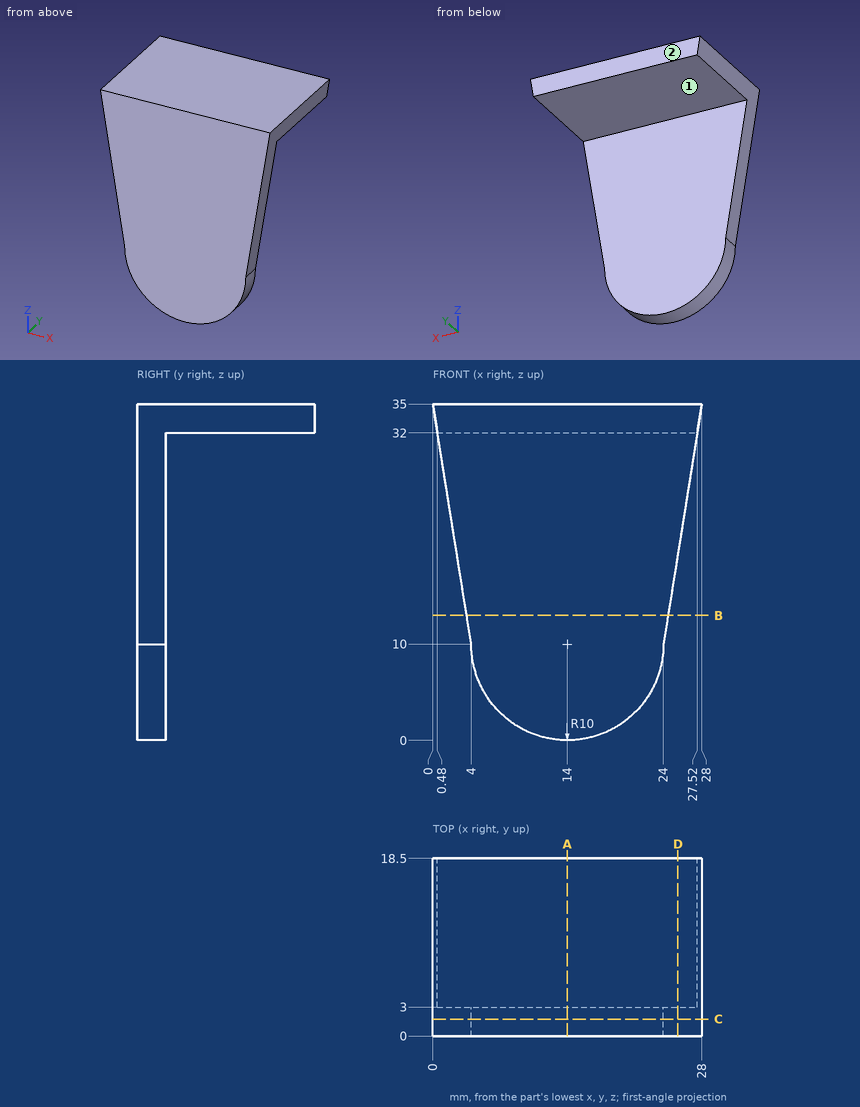
Source: three-view drawing plus pictorial views. Frame: mm from the lowest corner of the part. A direction names the side the tool comes from. Round coordinates to 2 decimals unless told otherwise and drop trailing zeros. Loops run counter-clockwise (first coordinate to the right, second up) from the corner with the lowest first, then second, coordinate; pieces in that order, holes last.
1. Ray query, L1, parallel to Z at x = 16.75, y = 5.75; L2, parallel to Y at x = 20.75, z = 3; L3, parallel to X at y = 1.75, z = 4.5. Return the intervals inside material, ascending.
2. Contact query for flat-ended pins moving along their axis: pin 1 (3 mm diameter, centred on x = 7, y = 6, fed in from -Z); pin 2 (8 mm diameter, centred on x = 12, z = 26.5, fed in from -Y); pin 3 (3 mm diameter, centred on x = 3.5, z = 19, fed in from +Y). Output: stop coordinate, or through.
3. Section query D-D on x = 25.5. Output: boundary loops of the cut face in (y, z) (3 decimals).
4. Access query for the marked faces 1 and 2. Directions: +Z, -Z, +X, -X, +Y, -Y. A direction counts if a zero-diameter tool reaches every point of the face in a straight line with its end or side. Return the directions, or none.
5. Section query B-B on z = 13. Output: boundary loops of the cut face in (x, y).
6. Section query A-A on x = 14. Output: boundary loops of the cut face in (y, z).
7. Section query C-C on y = 1.75. Output: boundary loops of the cut face in (x, z).
Answers below:
1. L1: z = 32 to 35
1. L2: y = 0 to 3
1. L3: x = 5.65 to 22.35
2. pin 1: stops at z = 32
2. pin 2: stops at y = 0
2. pin 3: stops at y = 3
3. outline: (0, 19.375) - (3, 19.375) - (3, 32) - (18.5, 32) - (18.5, 35) - (0, 35) - close
4. face 1: -Z, +X, -X, +Y
4. face 2: +Z, -Z, +X, -X, +Y
5. outline: (3.52, 0) - (24.48, 0) - (24.48, 3) - (3.52, 3) - close
6. outline: (0, 0) - (3, 0) - (3, 32) - (18.5, 32) - (18.5, 35) - (0, 35) - close
7. outline: (0, 35) - (4, 10) arc R10 ccw to (24, 10) - (28, 35) - close
